Verification items for the finished model (mm, model axes). A direction names the side the tool comes from. Round coordinates to 2 decimals unless told otherwise and drop trailing zeros. Write each loop counter-clockwise with the first axis right and the second up, starting at its lowest first coordinate (ties: lowest second). Pieces come first, ordered by that corner, then holes. Notation, with made-up numbers: M 36,88.25 L 93,88.25 A13 ccw 93,111.25 Z; hole C -5,-32 d5. An arc over 180 degrees is marked long. One line per item, written item: value. Start each with the question number.
Item 1: Gauge pin test, flat ends, axial feed: pin 1 (1.5 mm diameter, centred on y = 5, z = 1, fed in from +X); pin 2 (1.2 mm diameter, centred on y = 11.5, z = -1.5, fed in from +X). Record the tip position at first contact, or that the pin passes through.
Item 2: Draft check along Y on faces 1 (the face through (17, -2.5, 0)), 2 (the face through (-7.5, 5, 0)), 3 (the face through (-17, 2.5, 0)). Enter one of: +Y half, -Y half, draft (parallel to the pull), parting line (faces both ways), or undercut.
Item 3: Section check D-D, the plane z = 2.75. Record the cut outline in (x, y), then the cut area to 3 significant figures.
Item 4: Section check C-C, the plane y = 5. Record the cut outline in (x, z).
Item 5: Section check B-B, the plane x = -4. Record the cut outline in (y, z), then the cut area to 3 significant figures.
Item 6: Tool access check on faces 4 (the face through (17, 2.5, 0)), 5 (the face through (-15, 5, 0)), 6 (the face through (-15, 11, 0)). Record the directions out of +Z, -Z, +X, -X, +Y, -Y that give a thin tool (end or side, any length) a straight path to the whole face; none if there is none.
Item 7: Thickness scan on probe 1 along X at (y, z) = (10.7, 0); probe 2 along Z at (x, y) = (19, 11.1); probe 3 along X at (y, z) = (4.5, -1.5). Record the ranges inside material, lowest first. Write a range as from..to.
Item 8: Section check A-A, the plane y = -0.75. Record the cut outline in (x, z), then the cut area to 3 significant figures.
from build123d import *

# Parameters (mm, degrees)
SKETCH1_W            = 30
SKETCH1_H            = 7
BOSS_EXTRUDE1_DEPTH  = 10
SKETCH2_W            = 15
SKETCH2_H            = 4
CUT_EXTRUDE1_DEPTH   = 10
SKETCH3_R            = 1.75
CUT_EXTRUDE2_DEPTH   = 10
FILLET1_R            = 4
SKETCH4_W            = 7
SKETCH4_H            = 15
BOSS_EXTRUDE2_DEPTH  = 7
SKETCH5_W            = 7
SKETCH5_H            = 5
CUT_EXTRUDE3_DEPTH   = 7
SKETCH6_R            = 1.75
CUT_EXTRUDE4_DEPTH   = 16
FILLET2_R            = 3
FILLET2_OF_MIRROR1_R = 3


with BuildPart() as part:
    # Sketch1 → Boss-Extrude1 (new body)
    with BuildSketch(Plane(origin=(0, 0, 0), x_dir=(1, 0, 0), z_dir=(0, 1, 0))):
        Rectangle(SKETCH1_W, SKETCH1_H)
    extrude(amount=BOSS_EXTRUDE1_DEPTH)

    # Sketch2 → Cut-Extrude1 (cut)
    with BuildSketch(Plane(origin=(0, 10, 0), x_dir=(1, 0, 0), z_dir=(0, 1, 0))):
        Rectangle(SKETCH2_W, SKETCH2_H)
    extrude(amount=-CUT_EXTRUDE1_DEPTH, mode=Mode.SUBTRACT)

    # Sketch3 → Cut-Extrude2 (cut)
    with BuildSketch(Plane.XY.offset(3.5)):
        with Locations((0, 5)):
            Circle(SKETCH3_R)
    extrude(amount=-CUT_EXTRUDE2_DEPTH, mode=Mode.SUBTRACT)

    # Fillet1
    fillet1_edges = [part.edges().sort_by_distance(p)[0] for p in [
        (7.5, 0, 0),
        (-7.5, 0, 0),
        (7.5, 10, 0),
        (-7.5, 10, 0),
    ]]
    fillet(fillet1_edges, radius=FILLET1_R)

    # Sketch4 → Boss-Extrude2 (add)
    with BuildSketch(Plane(origin=(15, 0, 0), x_dir=(0, 0, -1), z_dir=(1, 0, 0))):
        with Locations((0, 5)):
            Rectangle(SKETCH4_W, SKETCH4_H)
    boss_extrude2 = extrude(amount=BOSS_EXTRUDE2_DEPTH)

    # Sketch5 → Cut-Extrude3 (cut)
    with BuildSketch(Plane(origin=(22, 0, 0), x_dir=(0, 0, -1), z_dir=(1, 0, 0))):
        with Locations((0, 5)):
            Rectangle(SKETCH5_W, SKETCH5_H)
    cut_extrude3 = extrude(amount=-CUT_EXTRUDE3_DEPTH, mode=Mode.SUBTRACT)

    # Sketch6 → Cut-Extrude4 (cut, through all)
    with BuildSketch(Plane(origin=(0, 12.5, 0), x_dir=(1, 0, 0), z_dir=(0, 1, 0))):
        with Locations((19, 0)):
            Circle(SKETCH6_R)
    cut_extrude4 = extrude(amount=-CUT_EXTRUDE4_DEPTH, mode=Mode.SUBTRACT)

    # Fillet2
    fillet2_edges = [part.edges().sort_by_distance(p)[0] for p in [
        (22, 0, -3.5),
        (22, 10, 3.5),
        (22, 10, -3.5),
        (22, 0, 3.5),
    ]]
    fillet(fillet2_edges, radius=FILLET2_R)

    # Mirror1: Boss-Extrude2, Cut-Extrude3, Cut-Extrude4 across plane
    add(boss_extrude2.mirror(Plane(origin=(0, 0, 0), x_dir=(0, 0, 1), z_dir=(1, 0, 0))))
    add(cut_extrude3.mirror(Plane(origin=(0, 0, 0), x_dir=(0, 0, 1), z_dir=(1, 0, 0))), mode=Mode.SUBTRACT)
    add(cut_extrude4.mirror(Plane(origin=(0, 0, 0), x_dir=(0, 0, 1), z_dir=(1, 0, 0))), mode=Mode.SUBTRACT)

    # Fillet2 of Mirror1
    fillet2_of_mirror1_edges = [part.edges().sort_by_distance(p)[0] for p in [
        (-22, 0, -3.5),
        (-22, 10, 3.5),
        (-22, 10, -3.5),
        (-22, 0, 3.5),
    ]]
    fillet(fillet2_of_mirror1_edges, radius=FILLET2_OF_MIRROR1_R)


solid = part.part
Response values:
1. pin 1: stops at x = 15
1. pin 2: stops at x = 21.97
2. face 1: -Y half
2. face 2: draft
2. face 3: undercut
3. outline: M -20.98,-2.5 L -15,-2.5 L -15,0 L 15,0 L 15,-2.5 L 20.98,-2.5 L 20.98,2.5 L 15,2.5 L 15,7.5 L 20.98,7.5 L 20.98,12.5 L 15,12.5 L 15,10 L -15,10 L -15,12.5 L -20.98,12.5 L -20.98,7.5 L -15,7.5 L -15,2.5 L -20.98,2.5 Z; hole C 0,5 d3.5
3. area: 410 mm2
4. outline: M -15,-3.5 L -1.75,-3.5 L -1.75,-2 L -7.5,-2 L -7.5,2 L -1.75,2 L -1.75,3.5 L -15,3.5 Z; M 1.75,-3.5 L 15,-3.5 L 15,3.5 L 1.75,3.5 L 1.75,2 L 7.5,2 L 7.5,-2 L 1.75,-2 Z
5. outline: M 0,-3.5 L 10,-3.5 L 10,-2 L 0,-2 Z; M 0,2 L 10,2 L 10,3.5 L 0,3.5 Z
5. area: 30.0 mm2
6. face 4: +Z, -Z, +X
6. face 5: +Z, -Z, -X
6. face 6: +Z, -Z, +Y
7. probe 1: x = -22..-20.75, -17.25..-15, 15..17.25, 20.75..22
7. probe 2: z = -3.5..-1.75, 1.75..3.5
7. probe 3: x = -15..-7.5, 7.5..15
8. outline: M -22,-0.5 A3 ccw -19,-3.5 L -15,-3.5 L -15,3.5 L -19,3.5 A3 ccw -22,0.5 Z; M 15,-3.5 L 19,-3.5 A3 ccw 22,-0.5 L 22,0.5 A3 ccw 19,3.5 L 15,3.5 Z; hole C -19,0 d3.5; hole C 19,0 d3.5
8. area: 71.0 mm2
